The figure shows three views and two pictorial views of one solid part (mm, origin at its lowest corner). Answer the questions. Coordinates: 2 decimals unless noted, no trailing zeros. Write each loop counter-clockwise with the first axis right and the second up, starting at its lowest first coordinate (ties: lowest second). Pieces come first, ordered by that corner, then holes.
Item 1: Determine the mould class of the marked faces 1, 2, 3 and 4 for opening direction X: released by +X, released by -X, zero draft, split by the parting line, or undercut.
Item 2: Straight lines are drawn through the part: probe 1 along Z at (x, y) = (46, 5.75); probe 2 along X at (y, z) = (8.5, 39.5) (1 decimal); probe 3 along X at (y, z) = (12, 38) (1 decimal). For each, find the intervals that lie inside material, in ascending order.
Item 3: Section D-D (y = 1.5) is taken. Give the vertices of the cut face in (x, z) (1 decimal), then the cut area to 3 significant figures.
Item 4: Section C-C (z = 11.5) is taken. Give the vertices of the cut face in (x, y).
Item 5: Section B-B (x = 46) is taken. Give the vertices of the cut face in (y, z).
Item 6: Each of these flat-tipped pins is pushed along its axis until it touches: P1, Ø3, axis at y = 17.5, z = 38, coming from the +X side; P2, Ø6, axis at x = 14, z = 76, coming from the +Y side; P3, Ø3, axis at y = 8, z = 65, coming from the -X side. Where does it stop, or does it pass through?
Item 7: Section A-A (y = 12.5) is taken. Give the vertices of the cut face in (x, z) (1 decimal).
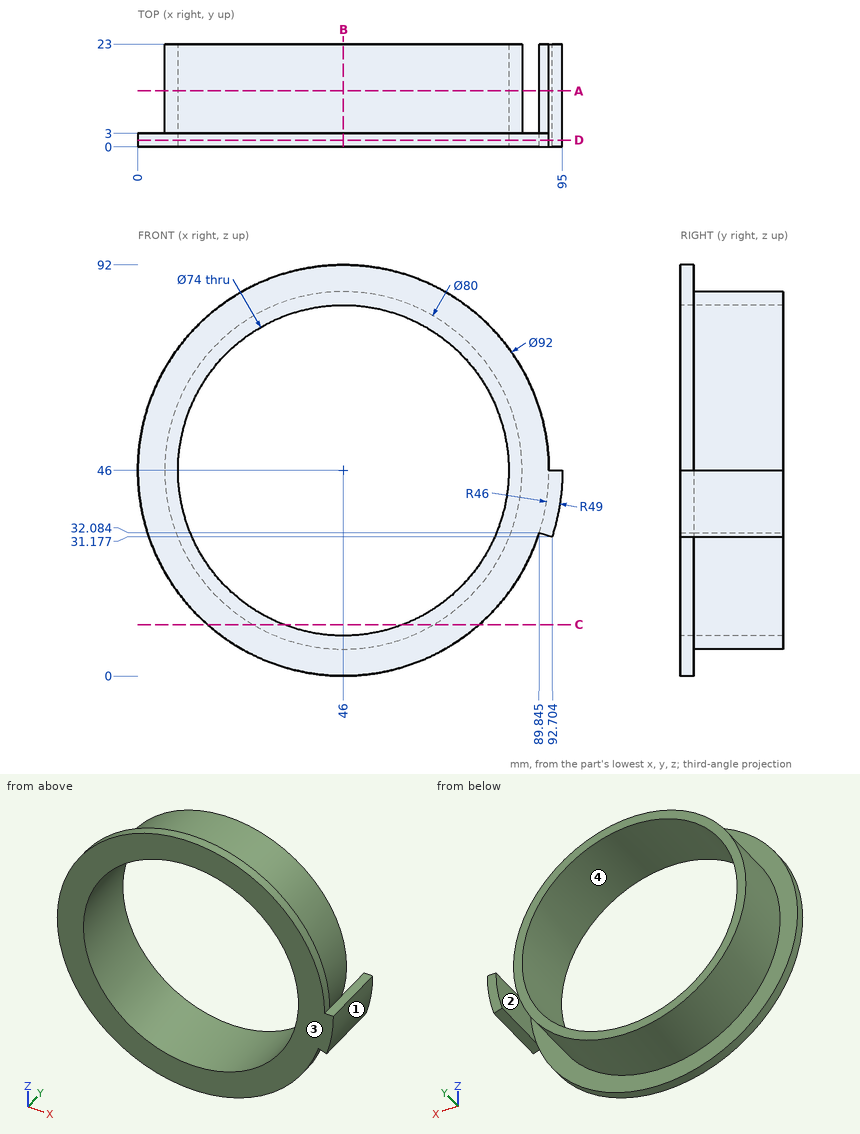
Established:
1. face 1: released by +X
1. face 2: undercut
1. face 3: zero draft
1. face 4: undercut
2. probe 1: z = 6 to 9, 83 to 86
2. probe 2: x = 6.5 to 9.6, 82.4 to 85.5, 91.5 to 94.6
2. probe 3: x = 6.8 to 9.9, 82.1 to 85.2, 91.3 to 94.3
3. outline: (89.8, 32.1) - (92.7, 31.2) arc R49 ccw to (95, 46) - (92, 46) arc R46 ccw (long way) to start; hole circle Ø74 at (46, 46)
3. area: 2,390 mm2
4. outline: (15.57, 0) - (32.63, 0) - (32.63, 23) - (25.76, 23) - (25.76, 3) - (15.57, 3) - close; (59.37, 0) - (76.43, 0) - (76.43, 3) - (66.24, 3) - (66.24, 23) - (59.37, 23) - close
5. outline: (0, 0) - (3, 0) - (3, 6) - (23, 6) - (23, 9) - (0, 9) - close; (0, 83) - (23, 83) - (23, 86) - (3, 86) - (3, 92) - (0, 92) - close
6. P1: stops at x = 94.57
6. P2: stops at y = 3
6. P3: stops at x = 10.03
7. outline: circle Ø80 at (46, 46); (89.8, 32.1) - (92.7, 31.2) arc R49 ccw to (95, 46) - (92, 46) arc R46 cw to start; hole circle Ø74 at (46, 46)
